The model under review builds one solid part; all positions refer to its coordinate system, in mm. A direction names the side the tool comes from. Round coordinates to 2 decimals unless told otherwise and drop trailing zeros. Order: outer loops, then holes, each group sorted by start corner. A loop starts at its lowest first (then second) coordinate and runs counter-clockwise, first axis right, second up.
```python
from build123d import *

# Parameters (mm, degrees)
SKETCH_2_R          = 3
EXTRUDE_1_DEPTH     = 16
SKETCH_6_R          = 4
EXTRUDE_2_DEPTH     = 4
FILLET_1_R          = 1
FILLET_2_R          = 0.5
CUT_EXTRUDE_1_DEPTH = 27.981475869
FILLET_3_R          = 4
SKETCH_8_R          = 1.25
CUT_EXTRUDE_2_DEPTH = 8


# Some blends are built 0.0001 mm under size
with BuildPart() as part:
    # 草图1 → 旋转1 (revolve)
    with BuildSketch(Plane.XY):
        with BuildLine():
            Line((0, 6), (0, -6))
            ThreePointArc((0, -6), (6, 0), (0, 6))
        make_face()
    revolve(axis=Axis((0, 6, 0), (0, -1, 0)))

    # 草图2 → 凸台-拉伸1 (add)
    with BuildSketch(Plane(origin=(0, 0, 0), x_dir=(0, 0, -1), z_dir=(1, 0, 0))):
        with Locations(Location((0, 0, 0), (0, 0, 180))):
            Circle(SKETCH_2_R)
    extrude(amount=EXTRUDE_1_DEPTH)

    # 草图4 → 切除-旋转1 (revolve, cut)
    with BuildSketch(Plane.XY):
        with BuildLine():
            Line((0, 6), (0, -6))
            ThreePointArc((0, -6), (-3.464101615, -4.898979486), (-5.656854249, -2))
            Line((-5.656854249, -2), (-3.464101615, -2))
            ThreePointArc((-3.464101615, -2), (-4, 0), (-3.464101615, 2))
            Line((-3.464101615, 2), (-5.656854249, 2))
            ThreePointArc((-5.656854249, 2), (-3.464101615, 4.898979486), (0, 6))
        make_face()
    revolve(axis=Axis((0, 13.897588957, 0), (0, -1, 0)), mode=Mode.SUBTRACT)

    # 草图6 → 凸台-拉伸2 (add)
    with BuildSketch(Plane(origin=(16, 0, 0), x_dir=(0, 0, -1), z_dir=(1, 0, 0))):
        Circle(SKETCH_6_R)
    extrude(amount=EXTRUDE_2_DEPTH)

    # 圆角1
    fillet_1_edges = [part.edges().sort_by_distance(p)[0] for p in [
        (16, 0, -3),
    ]]
    fillet(fillet_1_edges, radius=FILLET_1_R - 0.0001)  # a hair under: the kernel refuses the full size

    # 圆角2
    fillet_2_edges = [part.edges().sort_by_distance(p)[0] for p in [
        (16, 0, 4),
    ]]
    fillet(fillet_2_edges, radius=FILLET_2_R)

    # 草图7 → 切除-拉伸1 (cut, through all)
    with BuildSketch(Plane(origin=(20, 0, 0), x_dir=(0, 0, -1), z_dir=(1, 0, 0))):
        with BuildLine():
            Line((-2.645751311, 3), (2.645751311, 3))
            ThreePointArc((2.645751311, 3), (0, 4), (-2.645751311, 3))
        make_face()
        with BuildLine():
            Line((-2.645751311, -3), (2.645751311, -3))
            ThreePointArc((2.645751311, -3), (0, -4), (-2.645751311, -3))
        make_face()
    extrude(amount=-CUT_EXTRUDE_1_DEPTH, mode=Mode.SUBTRACT)

    # 圆角3
    # the kernel refuses this fillet: 4 mm, written as the material it adds along each edge
    with BuildSketch(Plane(origin=(5.196152423, 0, 0), x_dir=(0, 0.710521844411638, 0.7036751442348125), z_dir=(0, -0.7036751442348125, 0.710521844411638))) as fillet_3_piece_1_section:
        with BuildLine():
            CenterArc((7, -1.945276006), FILLET_3_R, 134.427004001, 45.572995999)
            ThreePointArc((4.2, 0.911295366), (3.628720823, 0.417827906), (3, 0))
            Line((3, 0), (3, -1.945276006))
        make_face()
    fillet_3_piece_1 = revolve(axis=Axis((5.196152423, 0, 0), (-1, 0, 0)), revolution_arc=269.445220203, mode=Mode.PRIVATE)
    fillet_3_piece_1 = split(fillet_3_piece_1, bisect_by=Plane(origin=(5.196152423, -2, 0), z_dir=(0, 1, 0)), keep=Keep.TOP, mode=Mode.PRIVATE)
    fillet_3_piece_1 = split(fillet_3_piece_1, bisect_by=Plane(origin=(5.196152423, 2, 0), z_dir=(0, -1, 0)), keep=Keep.TOP, mode=Mode.PRIVATE)
    add(fillet_3_piece_1)
    with BuildSketch(Plane(origin=(5.196152423, 0, 0), x_dir=(0, -0.7108184662614588, -0.7033755099672631), z_dir=(0, 0.7033755099672631, -0.7108184662614588))) as fillet_3_piece_2_section:
        with BuildLine():
            CenterArc((7, -1.945276006), FILLET_3_R, 134.427004001, 45.572995999)
            ThreePointArc((4.2, 0.911295366), (3.628720823, 0.417827906), (3, 0))
            Line((3, 0), (3, -1.945276006))
        make_face()
    fillet_3_piece_2 = revolve(axis=Axis((5.196152423, 0, 0), (-1, 0, 0)), revolution_arc=134.698452933, mode=Mode.PRIVATE)
    fillet_3_piece_2 = split(fillet_3_piece_2, bisect_by=Plane(origin=(5.196152423, -2, 0), z_dir=(0, 1, 0)), keep=Keep.TOP, mode=Mode.PRIVATE)
    add(fillet_3_piece_2)
    with BuildSketch(Plane(origin=(5.196152423, 0, 0), x_dir=(0, 0, 1), z_dir=(0, -1, 0))) as fillet_3_piece_3_section:
        with BuildLine():
            CenterArc((7, -1.945276006), FILLET_3_R, 134.427004001, 45.572995999)
            ThreePointArc((4.2, 0.911295366), (3.628720823, 0.417827906), (3, 0))
            Line((3, 0), (3, -1.945276006))
        make_face()
    fillet_3_piece_3 = revolve(axis=Axis((5.196152423, 0, 0), (-1, 0, 0)), revolution_arc=134.698452933, mode=Mode.PRIVATE)
    fillet_3_piece_3 = split(fillet_3_piece_3, bisect_by=Plane(origin=(5.196152423, 2, 0), z_dir=(0, -1, 0)), keep=Keep.TOP, mode=Mode.PRIVATE)
    add(fillet_3_piece_3)

    # 草图8 → 切除-拉伸2 (cut)
    with BuildSketch(Plane(origin=(20, 0, 0), x_dir=(0, 0, -1), z_dir=(1, 0, 0))):
        Circle(SKETCH_8_R)
    extrude(amount=-CUT_EXTRUDE_2_DEPTH, mode=Mode.SUBTRACT)


solid = part.part
```
(1) For faces 1 (the cylindrical face through (10, -3, 0)), 2 (the cylindrical face through (18, 0, 4)), 3 (the cylindrical face through (18, 0, -4)), 4 (the flat face through (12, 0, 0)), list the 3-axis set-ups (+Z, -Z, +X, -X, +Y, -Y) from which the entire face can be reached by the end or side of a thin tool; tool diameter is ignored.
Data:
face 1: none
face 2: +Z, +X
face 3: -Z, +X
face 4: +X
(2) Consider section A-A (x = -0.5). Write out the cut boundary in (y, z).
Data:
outline: (-2, -5.63) arc R5.98 ccw to (2, -5.63) - (2, -3.43) arc R3.97 cw to (-2, -3.43) - close; (-2, 3.43) arc R3.97 cw to (2, 3.43) - (2, 5.63) arc R5.98 ccw to (-2, 5.63) - close
(3) Consider section B-B (z = 5). Write out the cut boundary in (x, y), and give its area (3 significant figures).
Data:
outline: (-2.65, -2) - (2.65, -2) arc R3.32 ccw to (2.65, 2) - (-2.65, 2) arc R3.32 ccw to start
area: 24.8 mm2
(4) To check wall thickness, follow probe 1 along Y at (x, z) = (14.25, 0); probe 2 along Y at (x, z) = (5.5, 0.75); probe 3 along Y at (x, z) = (13, 2). State the ranges of each line that lie inside material, in increasing order.
Data:
probe 1: y = -3 to -1.25, 1.25 to 3
probe 2: y = -2.9 to -2.28, -2 to 2, 2.28 to 2.9
probe 3: y = -2.24 to 2.24
(5) Consider section C-C (x = 11). Write out the cut boundary in (y, z), and give its area (3 significant figures).
Data:
outline: circle Ø6 at (0, 0)
area: 28.3 mm2
(6) Insertion check: pin 1 (1.2 mm diameter, centred on y = 0, z = -0.5, fed in from +X); pin 2 (3.5 mm diameter, centred on x = -2, z = -1.5, fed in from +Y); pin 3 (1 mm diameter, centred on x = 1, y = -1, fed in from +Z). Each pin has a flat end and moves straight along its axis. Give the tip position at first contact, or say it passes through.
Data:
pin 1: stops at x = 12
pin 2: stops at y = 2
pin 3: stops at z = 5.93
(7) Draft analysis for pull direction Y (two halves, no side actions). For faces 5 (the cylindrical face through (16.06, -1.22, 0.27)), 6 (the flat face through (20, 1.4, 0.1)), 7 (the flat face through (18, -3, 0)), state which applies: pulls with the +Y half, pulls with the -Y half, needs draft (parallel to the pull), parting line crosses it, or undercut.
Data:
face 5: undercut
face 6: needs draft
face 7: pulls with the -Y half
